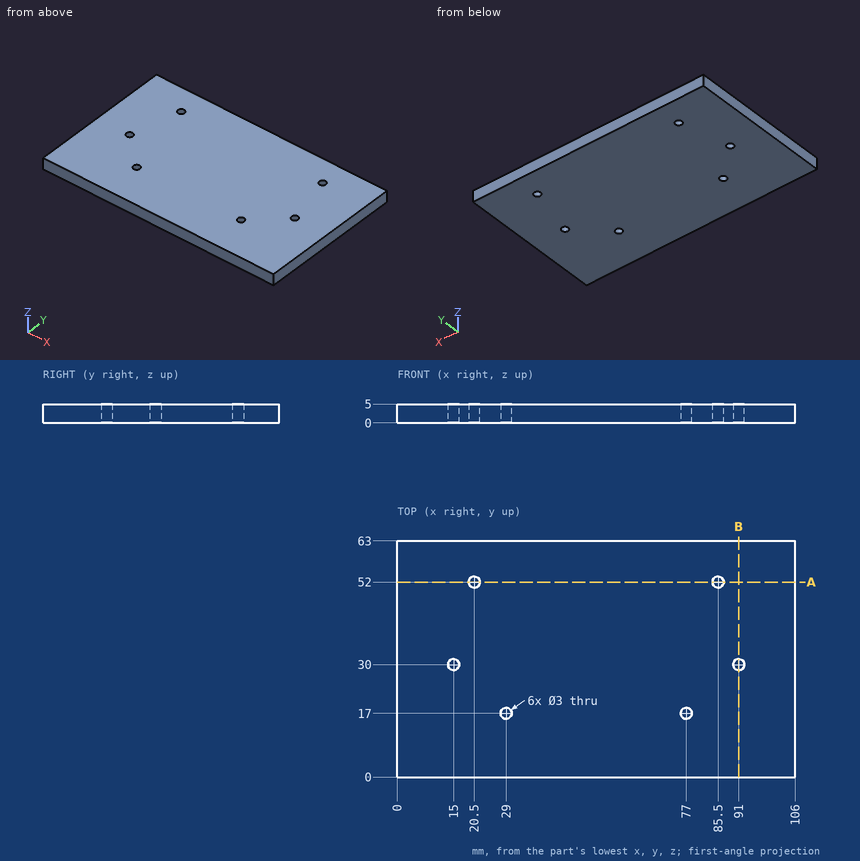
Geometry check sheet. Reference: drawing and pictorial views, mm from the part's lowest x, y, z. Coordinates: 2 decimals unless noted, no trailing zeros. Order: outer loops, then holes, each group sorted by start corner. A loop starts at its lowest first (then second) coordinate and runs counter-clockwise, first axis right, second up. Notation, with made-up numbers: (1.5, -6.5) -> (20.5, -6.5) arc R11 ccw to (20.5, -0.5) -> close; hole circle Ø2 at (72, -13). An arc over 180 degrees is marked (long way). Use CSV: the item, a comma, the result in double quotes. Start each with the question number.
Q1. Thickness scan on line 1 along X through (y, z) = (16.5, 4.5); line 2 along Y through (x, z) = (15, 2.3); line 3 along Y through (x, z) = (85.5, 3.6). Record the ranges inside material, lowest first.
Q2. Section check B-B, the plane x = 91. Record the cut outline in (y, z).
Q3. Section check A-A, the plane y = 52. Record the cut outline in (x, z), and give its area (3 significant figures).
Q4. Depth check by flat-ended pin: P1, Ø2.5, axis at x = 77, y = 17, coming from the -Z side. Enter the tip coordinate at first touch or a pass-through.
Returned:
1,line 1,"x = 0 to 27.59, 30.41 to 75.59, 78.41 to 106"
1,line 2,"y = 0 to 28.5, 31.5 to 63"
1,line 3,"y = 0 to 50.5, 53.5 to 63"
2,outline,"(0, 0) -> (28.5, 0) -> (28.5, 5) -> (0, 5) -> close; (31.5, 0) -> (63, 0) -> (63, 5) -> (31.5, 5) -> close"
3,outline,"(0, 0) -> (19, 0) -> (19, 5) -> (0, 5) -> close; (22, 0) -> (84, 0) -> (84, 5) -> (22, 5) -> close; (87, 0) -> (106, 0) -> (106, 5) -> (87, 5) -> close"
3,area,"500 mm^2"
4,P1,"passes through"
